Can you work these out from the model? Positions are in its coordinate system, mm. A direction names the side the tool comes from. Round coordinates to 2 decimals unless told otherwise and drop trailing zeros. Write each loop counter-clockwise with the first axis right and the second up, starting at its lowest first coordinate (ties: lowest second). Pieces come first, ordered by that corner, then holes.
Q1. If we section it at C-C (y = 4): Give the number of separate pieces and of enclosed holes in the cut face, plus the area to 3 significant figures.
Q2. I'm going to push flat-ended pins straight in: pin 1 Ø4 at (x, y) = (11.5, 3) entering from +Z; pin 2 Ø2 at (y, z) = (3.5, -23.5) entering from +X; pin 3 Ø1.3 at (x, z) = (0.5, -21.5) entering from -Y; pin 4 Ø4 at (y, z) = (-0.5, 15) entering from -X. Where does each tip first touch, or does it pass through?
Q3. For faces 3 (the cylindrical face through (20.16, 3.48, -8.09)), 4 (the cylindrical face through (0.1, 3.7, 16.9)), 5 (the cylindrical face through (10.726, -1.042, 17.351)), which set-ups out of +Z, -Z, +X, -X, +Y, -Y let a thin tool reach every point of the face, with its end or its side?
Q4. If we section it at A-A (z = 0): Please give me the cut outline in (x, y) (3 decimals).
Q5. We'd pull the mould along X, two halves only. Please class faces 1 (the cylindrical face through (-6.39, 4.01, -0.26)), 2 (the flat face through (-6, 5, 0)): +X half, -X half, draft (parallel to the pull), parting line (faces both ways), or undercut.
Q6. If we section it at B-B (z = -22): Please give me the cut outline in (x, y).
Q7. Please list where these lines run through material, in increasing order: line 1 along Z through (x, y) = (-15, -1.25); line 2 along X through (y, z) = (3.5, 17.5); line 3 along Z through (x, y) = (2, 2.5).
from build123d import *

# Parameters (mm, degrees)
SKETCH_1_R               = 30
SKETCH_1_R_2             = 1.25
SKETCH_1_R_3             = 5.5
EXTRUDE_1_DEPTH          = 5
CUT_EXTRUDE_START        = 5
SKETCH_1_15_R            = 2
CUT_EXTRUDE_2_DEPTH      = 2
SKETCH_2_R               = 3.1
CUT_EXTRUDE_3_DEPTH      = 2.6
EXTRUDE_START            = 4
SKETCH_3_R               = 30
SKETCH_3_R_2             = 14
EXTRUDE_2_DEPTH          = 4
SKETCH_4_R               = 1.5
CUT_EXTRUDE_4_DEPTH      = 44.370496884
SKETCH_4_3_R             = 2.25
CUT_EXTRUDE_5_DEPTH      = 6
PATTERN_CIRCULAR_1_COUNT = 10


with BuildPart() as part:
    # 草图1 → 凸台-拉伸1 (new body)
    with BuildSketch(Plane(origin=(0, 0, 0), x_dir=(1, 0, 0), z_dir=(0, 1, 0))):
        with Locations(Location((0, 0, 0), (0, 0, 270))):
            Circle(SKETCH_1_R)
        with Locations(Location((-8.375, 0, 0), (0, 0, 270))):
            Circle(SKETCH_1_R_2, mode=Mode.SUBTRACT)
        with Locations(Location((8.375, 0, 0), (0, 0, 270))):
            Circle(SKETCH_1_R_2, mode=Mode.SUBTRACT)
        with Locations(Location((0, 10.9, 0), (0, 0, 270))):
            Circle(SKETCH_1_R_2, mode=Mode.SUBTRACT)
        with Locations(Location((0, 0, 0), (0, 0, 270))):
            Circle(SKETCH_1_R_3, mode=Mode.SUBTRACT)
    extrude(amount=EXTRUDE_1_DEPTH)

    # 草图1<15> → 切除-拉伸2 (cut)
    with BuildSketch(Plane(origin=(0, 0, 0), x_dir=(1, 0, 0), z_dir=(0, 1, 0)).offset(CUT_EXTRUDE_START)):
        with Locations(Location((-8.375, 0, 0), (0, 0, 270))):
            Circle(SKETCH_1_15_R)
        with Locations(Location((8.375, 0, 0), (0, 0, 270))):
            Circle(SKETCH_1_15_R)
        with Locations(Location((0, 10.9, 0), (0, 0, 270))):
            Circle(SKETCH_1_15_R)
    extrude(amount=-CUT_EXTRUDE_2_DEPTH, mode=Mode.SUBTRACT)

    # 草图2 → 切除-拉伸3 (cut)
    with BuildSketch(Plane(origin=(0, 5, 0), x_dir=(1, 0, 0), z_dir=(0, 1, 0))):
        with Locations(Location((0, -20, 0), (0, 0, 270))):
            Circle(SKETCH_2_R)
        with Locations(Location((-18.428493563, -15.375, 0), (0, 0, 270))):
            Circle(SKETCH_2_R)
    extrude(amount=-CUT_EXTRUDE_3_DEPTH, mode=Mode.SUBTRACT)

    # 草图3 → 凸台-拉伸2 (add)
    with BuildSketch(Plane.XZ.offset(EXTRUDE_START)):
        with Locations(Location((0, 0, 0), (0, 0, 270))):
            Circle(SKETCH_3_R)
        with Locations(Location((0, 0, 0), (0, 0, 270))):
            Circle(SKETCH_3_R_2, mode=Mode.SUBTRACT)
    extrude(amount=-EXTRUDE_2_DEPTH)

    # 草图4 → 切除-拉伸4 (cut, through all)
    with BuildSketch(Plane.XZ.offset(4)):
        with Locations(Location((0, -22, 0), (0, 0, 270))):
            Circle(SKETCH_4_R)
    cut_extrude_4 = extrude(amount=-CUT_EXTRUDE_4_DEPTH, mode=Mode.SUBTRACT)

    # 草图4<3> → 切除-拉伸5 (cut)
    with BuildSketch(Plane.XZ.offset(4)):
        with Locations(Location((0, -22, 0), (0, 0, 270))):
            Circle(SKETCH_4_3_R)
    cut_extrude_5 = extrude(amount=-CUT_EXTRUDE_5_DEPTH, mode=Mode.SUBTRACT)

    # 阵列(圆周)1: 切除-拉伸4, 切除-拉伸5 ×10 about axis
    pattern_circular_1_axis = Axis((0, 0, 0), (0, 1, 0))
    add([cut_extrude_4.rotate(pattern_circular_1_axis, i * 360 / PATTERN_CIRCULAR_1_COUNT) for i in range(1, PATTERN_CIRCULAR_1_COUNT)], mode=Mode.SUBTRACT)
    add([cut_extrude_5.rotate(pattern_circular_1_axis, i * 360 / PATTERN_CIRCULAR_1_COUNT) for i in range(1, PATTERN_CIRCULAR_1_COUNT)], mode=Mode.SUBTRACT)


solid = part.part
A:
1. separate pieces: 1
1. enclosed holes: 15
1. area: 2,570 mm2
2. pin 1: stops at z = 28.46
2. pin 2: stops at x = 19.84
2. pin 3: passes through
2. pin 4: stops at x = -27.04
3. face 3: +Y, -Y
3. face 4: +Y
3. face 5: -Y
4. outline: (-30, -4) - (-14, -4) - (-14, 0) - (-9.625, 0) - (-9.625, 3) - (-10.375, 3) - (-10.375, 5) - (-30, 5) - close; (-7.125, 0) - (-5.5, 0) - (-5.5, 5) - (-6.375, 5) - (-6.375, 3) - (-7.125, 3) - close; (5.5, 0) - (7.125, 0) - (7.125, 3) - (6.375, 3) - (6.375, 5) - (5.5, 5) - close; (9.625, 0) - (14, 0) - (14, -4) - (30, -4) - (30, 5) - (10.375, 5) - (10.375, 3) - (9.625, 3) - close
5. face 1: undercut
5. face 2: draft
6. outline: (-20.4, -4) - (-2.25, -4) - (-2.25, 2) - (-1.5, 2) - (-1.5, 5) - (-20.4, 5) - close; (1.5, 2) - (2.25, 2) - (2.25, -4) - (20.4, -4) - (20.4, 5) - (1.5, 5) - close
7. line 1: z = -25.98 to -18.68, -16.91 to 16.91, 18.68 to 25.98
7. line 2: x = -24.37 to -20.69, -16.17 to -14.4, -11.46 to -1.83, 1.83 to 11.46, 14.4 to 24.37
7. line 3: z = -29.93 to -5.12, 5.12 to 17.63, 22.37 to 29.93
